Job drawing, mm, ordinate dimensions from the low corner. One solid piece. A direction names the side the tool comes from. Round coordinates to 2 decimals unless told otherwise and drop trailing zeros. Write each loop counter-clockwise with the first axis right and the second up, starting at its lowest first coordinate (ties: lowest second). Pieces come first, ordered by that corner, then holes. Notation, with made-up numbers: M 49,65 L 61,65 A20 cw 61,80 Z; hole C 22.25,-22 d3. An arc over 180 degrees is marked long. One line per item, written item: value. Start each with the question number.
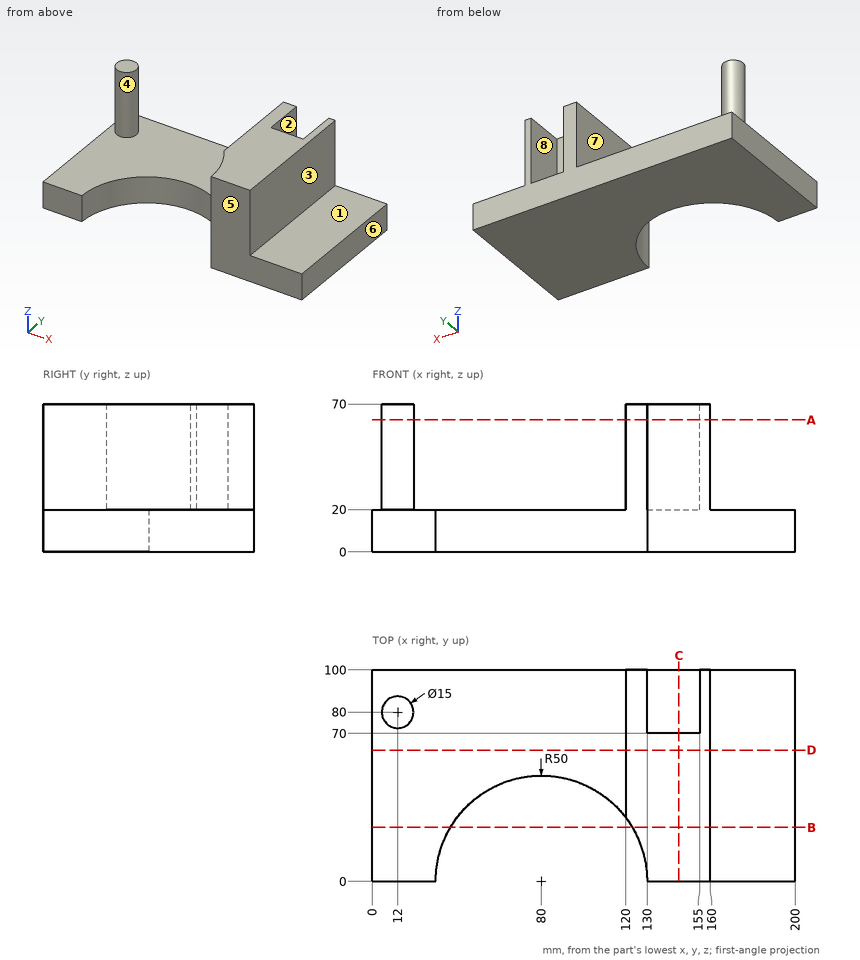
Item 1: Cut at A-A, the plane z = 62.5. Write the cut outline in (x, y).
Item 2: Which spindle directions (+Z, -Z, +X, -X, +Y, -Y) get a long thin tool onto all of the face, cutting with end or side? Do the marked faces 4, 5, 6, 7 and 8. Say none if no direction does.
Item 3: Cut at B-B, the plane y = 25.5. Write the cut outline in (x, z), plus the area to 3 significant figures.
Item 4: Cut at D-D, the plane y = 62. Write the cut outline in (x, z).
Item 5: Cut at C-C, the plane x = 145. Write the cut outline in (y, z), plus the area to 3 significant figures.
Item 6: Drill centre lines: line 1 (X direction, y = 78, z = 36); line 2 (Z direction, x = 161, y = 80); line 3 (X direction, y = 90, z = 25). Where is each one in solid material? Low to high.
Item 7: Drop flat-ended pins along their axis: pin 1 (15 mm diameter, centred on y = 82, z = 53.5, fed in from +X); pin 2 (8 mm diameter, centred on y = 20, z = 57, fed in from -X); pin 3 (6 mm diameter, centred on y = 48.5, z = 62.5, fed in from -X); pin 4 (1 mm diameter, centred on y = 22.5, z = 19.5, fed in from -X). Give the stop position or say it passes through.
Item 8: Two-plate mould, pull along X, no slides. Class the marked faces 1, 2 and 3: pulls with the +X half, pulls with the -X half, needs draft (parallel to the pull), parting line crosses it, or undercut.
Computed values:
1. outline: C 12,80 d15; M 120,30 A50 cw 130,0 L 160,0 L 160,100 L 155,100 L 155,70 L 130,70 L 130,100 L 120,100 Z
2. face 4: +Z
2. face 5: +Z, -Z, +X, -X, -Y
2. face 6: +Z, -Z, +X, +Y, -Y
2. face 7: +Z, +Y, -Y
2. face 8: +Z, +Y
3. outline: M 0,0 L 36.99,0 L 36.99,20 L 0,20 Z; M 123.01,0 L 200,0 L 200,20 L 160,20 L 160,70 L 123.01,70 Z
3. area: 4,130 mm2
4. outline: M 0,0 L 200,0 L 200,20 L 160,20 L 160,70 L 120,70 L 120,20 L 0,20 Z
5. outline: M 0,0 L 100,0 L 100,20 L 70,20 L 70,70 L 0,70 Z
5. area: 5,500 mm2
6. line 1: x = 4.77 to 19.23, 120 to 130, 155 to 160
6. line 2: z = 0 to 20
6. line 3: x = 120 to 130, 155 to 160
7. pin 1: stops at x = 160
7. pin 2: stops at x = 123.86
7. pin 3: stops at x = 120
7. pin 4: stops at x = 0
8. face 1: needs draft
8. face 2: undercut
8. face 3: pulls with the +X half
